```python
from build123d import *

# Parameters (mm, degrees)
SKETCH1_R           = 38.1
BOSS_EXTRUDE1_DEPTH = 6.35
SKETCH2_R           = 25.4
BOSS_EXTRUDE2_DEPTH = 25.4
SKETCH3_R           = 47.625
SKETCH3_R_2         = 38.1
BOSS_EXTRUDE3_DEPTH = 12.7
CUT_EXTRUDE3_DEPTH  = 32.75
BOSS_EXTRUDE4_DEPTH = 6.35


with BuildPart() as part:
    # Sketch1 → Boss-Extrude1 (new body)
    with BuildSketch(Plane(origin=(0, 0, 0), x_dir=(1, 0, 0), z_dir=(0, 1, 0))):
        Circle(SKETCH1_R)
    extrude(amount=BOSS_EXTRUDE1_DEPTH)

    # Sketch2 → Boss-Extrude2 (add)
    with BuildSketch(Plane(origin=(0, 6.35, 0), x_dir=(1, 0, 0), z_dir=(0, 1, 0))):
        Circle(SKETCH2_R)
    extrude(amount=BOSS_EXTRUDE2_DEPTH)

    # Sketch3 → Boss-Extrude3 (add)
    with BuildSketch(Plane(origin=(0, 0, 0), x_dir=(1, 0, 0), z_dir=(0, 1, 0))):
        Circle(SKETCH3_R)
        Circle(SKETCH3_R_2, mode=Mode.SUBTRACT)
    extrude(amount=BOSS_EXTRUDE3_DEPTH)

    # Sketch4 → Cut-Extrude3 (cut, through all)
    with BuildSketch(Plane(origin=(0, 0, 0), x_dir=(1, 0, 0), z_dir=(0, 1, 0))):
        Polygon((-18.8595, -13.731963353), (18.8595, -13.731963353), (18.8595, -50.573816251), (47.625, -50.573816251), (47.625, 47.625), (19.007906819, 47.625), (-18.8595, 47.625), (-47.625, 47.625), (-47.625, -44.321865457), (-18.8595, -44.321865457), align=None)
    extrude(amount=CUT_EXTRUDE3_DEPTH, mode=Mode.SUBTRACT)

    # Sketch5 → Boss-Extrude4 (add)
    with BuildSketch(Plane(origin=(0, 12.7, 0), x_dir=(1, 0, 0), z_dir=(0, 1, 0))):
        with BuildLine():
            Line((-9.398, -44.45), (9.398, -44.45))
            Line((9.398, -44.45), (9.398, -36.922724656))
            ThreePointArc((9.398, -36.922724656), (0, -38.1), (-9.398, -36.922724656))
            Line((-9.398, -36.922724656), (-9.398, -44.45))
        make_face()
    extrude(amount=BOSS_EXTRUDE4_DEPTH)


solid = part.part
```
Here's how the part is built. I have some questions about the finished solid (model axes, mm). A direction names the side the tool comes from. Round coordinates to 2 decimals unless told otherwise and drop trailing zeros. Write each loop counter-clockwise with the first axis right and the second up, starting at its lowest first coordinate (ties: lowest second). Pieces come first, ordered by that corner, then holes.
Q1. Please list where these lines run through material, in increasing order: probe 1 along Y at (x, z) = (-15.5, 38); probe 2 along Z at (x, y) = (-1.5, 12); probe 3 along Y at (x, z) = (-4.5, 25.5).
Q2. If we section it at B-B on x = 0: Write out the boundary of the cut face in (y, z) (3 decimals), plus the area to 3 significant figures.
Q3. Will these pins go through, and if not, where does the flat tip stop? P1, Ø8, axis at x = -5, y = 15, coming from the +Z side; P2, Ø5, axis at y = 15, z = 40, coming from the -X side; P3, Ø3, axis at y = 14.5, z = 40.5, coming from the +X side; P4, Ø1.9, axis at x = 3.5, y = 14.5, coming from the +Z side.
Q4. Which directions (+Z, -Z, +X, -X, +Y, -Y) give clear straight access to the entire face, cutting with the end or side of a thin tool? Please do faces 1 (the flat face through (0, 16, 44.45)), 2 (the flat face through (9.398, 16, 41)), 3 (the flat face through (-18.86, 5, 29)), 4 (the cylindrical face through (-0.3, 18.9, 25.4)).
Q5. If we section it at A-A on y = 13.5: Write out the boundary of the cut face in (x, z).
Q6. If we mould it in two halves opening along X, with no side actions, what happens to faces 5 (the cylindrical face through (-0.271, 6.261, 47.624)), 6 (the flat face through (0, 6.35, 30)), 7 (the flat face through (-9.398, 16, 41))? For each: +X half, -X half, draft (parallel to the pull), parting line (faces both ways), or undercut.
Q7. If we section it at C-C on z = 20.5: Write out the boundary of the cut face in (x, y), plus the area to 3 significant figures.
Answer below:
1. probe 1: y = 0 to 12.7
1. probe 2: z = 13.73 to 25.36, 38.07 to 47.6
1. probe 3: y = 0 to 6.35
2. outline: (0, 13.732) - (31.75, 13.732) - (31.75, 25.4) - (6.35, 25.4) - (6.35, 38.1) - (19.05, 38.1) - (19.05, 44.45) - (12.7, 44.45) - (12.7, 47.625) - (0, 47.625) - close
2. area: 612 mm2
3. P1: stops at z = 47.59
3. P2: stops at x = -18.86
3. P3: stops at x = 9.4
3. P4: stops at z = 44.45
4. face 1: +Z, +X, -X, +Y
4. face 2: +Z, +X, +Y
4. face 3: +Z, -Z, -X, +Y, -Y
4. face 4: +Y
5. outline: (-18.86, 13.73) - (18.86, 13.73) - (18.86, 17.01) arc R25.4 ccw to (-18.86, 17.01) - close; (-9.4, 36.92) arc R38.1 cw to (9.4, 36.92) - (9.4, 44.45) - (-9.4, 44.45) - close
6. face 5: parting line
6. face 6: undercut
6. face 7: -X half
7. outline: (-18.86, 0) - (18.86, 0) - (18.86, 6.35) - (15, 6.35) - (15, 31.75) - (-15, 31.75) - (-15, 6.35) - (-18.86, 6.35) - close
7. area: 1,000 mm2
